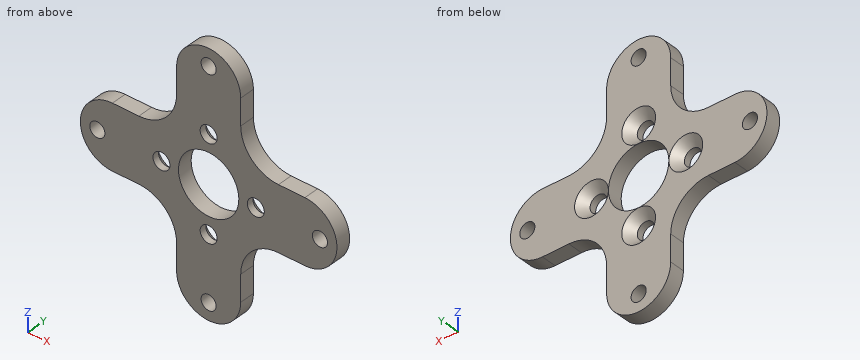
from build123d import *

# Parameters (mm, degrees)
ESBO_O1_W                           = 17
ESBO_O1_H                           = 17
RESSALTO_EXTRUS_O1_DEPTH            = 2
FILETE1_R                           = 10
ESBO_O3_R                           = 8
ESBO_O3_R_2                         = 2
CORTE_EXTRUS_O1_DEPTH               = 49.249352327
PADR_OCIRCULAR1_COUNT               = 4
ESCAREADO_PARA_SFHCS_M41_AT_2_COUNT = 2
ESCAREADO_PARA_SFHCS_M41_AT_2_PITCH = 17.67766953
ESCAREADO_PARA_SFHCS_M41_AT_3_COUNT = 2
ESCAREADO_PARA_SFHCS_M41_AT_3_PITCH = 25
ESCAREADO_PARA_SFHCS_M41_AT_4_COUNT = 2
ESCAREADO_PARA_SFHCS_M41_AT_4_PITCH = 17.67766953


with BuildPart() as part:
    # Esboço1 → Ressalto-extrusão1 (new, symmetric)
    with BuildSketch(Plane(origin=(0, 0, 0), x_dir=(1, 0, 0), z_dir=(0, 1, 0))):
        with BuildLine():
            Line((-8.5, -8.5), (-8.5, 8.5))
            Line((-8.5, 8.5), (-25.5, 8.5))
            ThreePointArc((-25.5, 8.5), (-34, 0), (-25.5, -8.5))
            Line((-25.5, -8.5), (-8.5, -8.5))
        make_face()
        with BuildLine():
            Line((8.5, 8.5), (8.5, 25.5))
            ThreePointArc((8.5, 25.5), (0, 34), (-8.5, 25.5))
            Line((-8.5, 25.5), (-8.5, 8.5))
            Line((-8.5, 8.5), (8.5, 8.5))
        make_face()
        Rectangle(ESBO_O1_W, ESBO_O1_H)
        with BuildLine():
            Line((25.5, 8.5), (8.5, 8.5))
            Line((8.5, 8.5), (8.5, -8.5))
            Line((8.5, -8.5), (25.5, -8.5))
            ThreePointArc((25.5, -8.5), (34, 0), (25.5, 8.5))
        make_face()
        with BuildLine():
            Line((8.5, -25.5), (8.5, -8.5))
            Line((8.5, -8.5), (-8.5, -8.5))
            Line((-8.5, -8.5), (-8.5, -25.5))
            ThreePointArc((-8.5, -25.5), (0, -34), (8.5, -25.5))
        make_face()
    extrude(amount=RESSALTO_EXTRUS_O1_DEPTH, both=True)

    # Filete1
    filete1_edges = [part.edges().sort_by_distance(p)[0] for p in [
        (-8.5, 0, -8.5),
        (8.5, 0, -8.5),
        (8.5, 0, 8.5),
        (-8.5, 0, 8.5),
    ]]
    fillet(filete1_edges, radius=FILETE1_R)

    # Esboço3 → Corte-extrusão1 (cut, through all)
    with BuildSketch(Plane(origin=(0, 2, 0), x_dir=(1, 0, 0), z_dir=(0, 1, 0))):
        with Locations(Location((0, 0, 0), (0, 0, 270))):
            Circle(ESBO_O3_R)
        with Locations(Location((0, 29.5, 0), (0, 0, 270))):
            Circle(ESBO_O3_R_2)
    corte_extrus_o1 = extrude(amount=-CORTE_EXTRUS_O1_DEPTH, mode=Mode.SUBTRACT)

    # PadrãoCircular1: Corte-extrusão1 ×4 about axis
    padr_ocircular1_axis = Axis((0, 0, 0), (0, 1, 0))
    for i in range(1, PADR_OCIRCULAR1_COUNT):
        add(corte_extrus_o1.rotate(padr_ocircular1_axis, i * 360 / PADR_OCIRCULAR1_COUNT), mode=Mode.SUBTRACT)

    # Esboço6 → Escareado para SFHCS M41 (revolve, cut)
    with BuildSketch(Plane(origin=(-12.5, 2, 0), x_dir=(0, 0, 1), z_dir=(1, 0, 0))):
        Polygon((0, 0), (0, 4), (2.25, 4), (2.25, 2.23), (4.48, 0), align=None)
    escareado_para_sfhcs_m41 = revolve(axis=Axis((-12.5, 8.35, 0), (0, -1, 0)), mode=Mode.SUBTRACT)

    # Escareado para SFHCS M41 at 2: Escareado para SFHCS M41 ×2
    with Locations(*[Vector(0.7071067811865476, 0, -0.7071067811865476) * (i * ESCAREADO_PARA_SFHCS_M41_AT_2_PITCH) for i in range(1, ESCAREADO_PARA_SFHCS_M41_AT_2_COUNT)]):
        add(escareado_para_sfhcs_m41, mode=Mode.SUBTRACT)

    # Escareado para SFHCS M41 at 3: Escareado para SFHCS M41 ×2
    with Locations(*[(i * ESCAREADO_PARA_SFHCS_M41_AT_3_PITCH, 0, 0) for i in range(1, ESCAREADO_PARA_SFHCS_M41_AT_3_COUNT)]):
        add(escareado_para_sfhcs_m41, mode=Mode.SUBTRACT)

    # Escareado para SFHCS M41 at 4: Escareado para SFHCS M41 ×2
    with Locations(*[Vector(0.7071067811865476, 0, 0.7071067811865476) * (i * ESCAREADO_PARA_SFHCS_M41_AT_4_PITCH) for i in range(1, ESCAREADO_PARA_SFHCS_M41_AT_4_COUNT)]):
        add(escareado_para_sfhcs_m41, mode=Mode.SUBTRACT)


solid = part.part
For this review, take the finished solid that the model builds, in its own axes (mm). Give positions to 0.01 mm unless a question says otherwise; leave off trailing zeros. Loops run counter-clockwise (first coordinate to the right, second up) from the corner with the lowest first, then second, coordinate; pieces in that order, holes last. Notation, with made-up numbers: M -26.75,-28 L 25.25,-28 A16 ccw 25.25,-9 Z; hole C 78,47.5 d11. An arc over 180 degrees is marked long. Put each result on its own line as item: value. Start each with the question number.
(1) Wall thickness on L1, parallel to X at y = 0.15, z = 31; L2, parallel to X at y = 0.4, z = -29.5; L3, parallel to X at y = -0.65, z = -26: over which ranges is each line inside the solid? List them lowest first.
(2) Add section A-A, the plane z = -29.5. Write out the cut boundary in (x, y).
(3) Add section D-D, the plane x = -29.5. Write out the cut boundary in (y, z).
(4) Add section C-C, the plane y = -0.95. Give the number of separate pieces and of enclosed holes in the cut face, then the cut area to 3 significant figures.
(5) For pin 1 (1.2 mm diameter, centred on y = 1, z = 21.5, fed in from -X); pin 2 (1.2 mm diameter, centred on x = 23, y = 0, fed in from -Z); pin 3 (2.5 mm diameter, centred on x = -12.5, z = 0, fed in from +Y); pin 4 (1 mm diameter, centred on x = -11.5, y = 1.5, fed in from -Z), all flat-tipped, find the tip position at first contact; note any pin that passes through.
(6) Add section B-B, the plane x = -12.5. Write out the cut boundary in (y, z).
Result:
1. L1: x = -6.48 to -1.32, 1.32 to 6.48
1. L2: x = -7.5 to -2, 2 to 7.5
1. L3: x = -8.49 to 8.49
2. outline: M -7.5,-2 L -2,-2 L -2,2 L -7.5,2 Z; M 2,-2 L 7.5,-2 L 7.5,2 L 2,2 Z
3. outline: M -2,-7.5 L 2,-7.5 L 2,-2 L -2,-2 Z; M -2,2 L 2,2 L 2,7.5 L -2,7.5 Z
4. separate pieces: 1
4. enclosed holes: 9
4. area: 1,670 mm^2
5. pin 1: stops at x = -8.5
5. pin 2: stops at z = -8.5
5. pin 3: passes through
5. pin 4: stops at z = -11.89
6. outline: M -2,-10.5 L 2,-10.5 L 2,-4.48 L -0.23,-2.25 L -2,-2.25 Z; M -2,2.25 L -0.23,2.25 L 2,4.48 L 2,10.5 L -2,10.5 Z
